```python
from build123d import *

# Parameters (mm, degrees)
F0_W     = 15.5
F0_H     = 15.5
F0_W_2   = 96
F0_H_2   = 44
F1_DEPTH = 5
F3_DEPTH = 5


with BuildPart() as f1:
    # F0 (on Top) → F1 (new body)
    with BuildSketch(Plane.XY):
        with BuildLine():
            ThreePointArc((0, 5), (1.464466, 1.464466), (5, 0))
            Line((5, 0), (105, 0))
            ThreePointArc((105, 0), (108.535534, 1.464466), (110, 5))
            Line((110, 5), (110, 170))
            ThreePointArc((110, 170), (108.535534, 173.535534), (105, 175))
            Line((105, 175), (5, 175))
            ThreePointArc((5, 175), (1.464466, 173.535534), (0, 170))
            Line((0, 170), (0, 5))
        make_face()
        with Locations((16.75, 16.75)):
            Rectangle(F0_W, F0_H, mode=Mode.SUBTRACT)
        with Locations((16.75, 42.25)):
            Rectangle(F0_W, F0_H, mode=Mode.SUBTRACT)
        with Locations((42.25, 16.75)):
            Rectangle(F0_W, F0_H, mode=Mode.SUBTRACT)
        with Locations((42.25, 42.25)):
            Rectangle(F0_W, F0_H, mode=Mode.SUBTRACT)
        with Locations((16.75, 67.75)):
            Rectangle(F0_W, F0_H, mode=Mode.SUBTRACT)
        with Locations((42.25, 67.75)):
            Rectangle(F0_W, F0_H, mode=Mode.SUBTRACT)
        with Locations((67.75, 16.75)):
            Rectangle(F0_W, F0_H, mode=Mode.SUBTRACT)
        with Locations((67.75, 42.25)):
            Rectangle(F0_W, F0_H, mode=Mode.SUBTRACT)
        with Locations((93.25, 16.75)):
            Rectangle(F0_W, F0_H, mode=Mode.SUBTRACT)
        with Locations((93.25, 42.25)):
            Rectangle(F0_W, F0_H, mode=Mode.SUBTRACT)
        with Locations((67.75, 67.75)):
            Rectangle(F0_W, F0_H, mode=Mode.SUBTRACT)
        with Locations((93.25, 67.75)):
            Rectangle(F0_W, F0_H, mode=Mode.SUBTRACT)
        with Locations((16.75, 93.25)):
            Rectangle(F0_W, F0_H, mode=Mode.SUBTRACT)
        with Locations((42.25, 93.25)):
            Rectangle(F0_W, F0_H, mode=Mode.SUBTRACT)
        with Locations((67.75, 93.25)):
            Rectangle(F0_W, F0_H, mode=Mode.SUBTRACT)
        with Locations((93.25, 93.25)):
            Rectangle(F0_W, F0_H, mode=Mode.SUBTRACT)
        with Locations((55, 138)):
            Rectangle(F0_W_2, F0_H_2, mode=Mode.SUBTRACT)
    extrude(amount=F1_DEPTH)

    # F2 (on face) → F3 (join)
    with BuildSketch(Plane.XY):
        with BuildLine():
            ThreePointArc((108, 168), (106.535534, 171.535534), (103, 173))
            Line((103, 173), (7, 173))
            ThreePointArc((7, 173), (3.464466, 171.535534), (2, 168))
            Line((2, 168), (2, 7))
            ThreePointArc((2, 7), (3.464466, 3.464466), (7, 2))
            Line((7, 2), (103, 2))
            ThreePointArc((103, 2), (106.535534, 3.464466), (108, 7))
            Line((108, 7), (108, 168))
        make_face()
        with BuildLine():
            Line((8, 172), (102, 172))
            ThreePointArc((102, 172), (105.535534, 170.535534), (107, 167))
            Line((107, 167), (107, 8))
            ThreePointArc((107, 8), (105.535534, 4.464466), (102, 3))
            Line((102, 3), (8, 3))
            ThreePointArc((8, 3), (4.464466, 4.464466), (3, 8))
            Line((3, 8), (3, 167))
            ThreePointArc((3, 167), (4.464466, 170.535534), (8, 172))
        make_face(mode=Mode.SUBTRACT)
    extrude(amount=-F3_DEPTH)


solid = f1.part
```
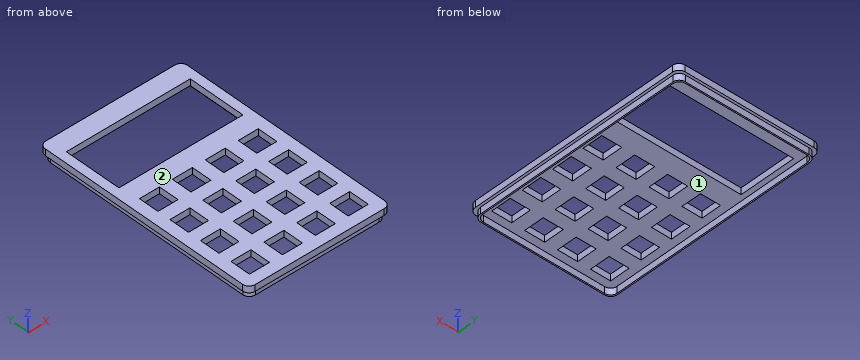
Source: CAD feature listing. Evaluate the final solid. Frame: model axes, mm. Face numbers are marked on the shaded views. Give positions to 0.01 mm unless a question says otherwise; leave off trailing zeros. Order: outer loops, then holes, each group sorted by start corner. A loop starts at its lowest first (then second) coordinate and runs counter-clockwise, first axis right, second up.
(1) Section query A-A (x = 30.5). Return the cut outline in (y, z).
(2) Section query D-D (y = 45). Return the cut outline in (x, z).
(3) Section query C-C (x = 67.5). State how many separate pieces and enclosed holes the cut face has, plus the area to 3 significant figures.
(4) Section query B-B (y = 151). Return the cut outline in (x, z), plus the area to 3 significant figures.
(5) Pull-direction query (X, two-part tool) for the marked faces 1 and 2; classes: +X half, -X half, draft (parallel to the pull), parting line (faces both ways), or undercut.
(6) Material intervals for line 1 along X through (y, z) = (96, 3.75); line 2 along Y through (x, z) = (68, 1.5); line 3 along X through (y, z) = (67, -4.5), sorted ascending.
(7) Contact query for flat-ended pins moving along their axis: P1, Ø1.5, axis at x = 38, y = 78, coming from the -Z side; P2, Ø4, axis at x = 98, y = 41.5, coming from the -Z side; P3, Ø1.5, axis at y = 56, z = -3.5, coming from the +X side. Output: stop coordinate, or through.
Outcome:
1. outline: (0, 0) - (2, 0) - (2, -5) - (3, -5) - (3, 0) - (116, 0) - (116, 5) - (0, 5) - close; (160, 0) - (172, 0) - (172, -5) - (173, -5) - (173, 0) - (175, 0) - (175, 5) - (160, 5) - close
2. outline: (0, 0) - (2, 0) - (2, -5) - (3, -5) - (3, 0) - (9, 0) - (9, 5) - (0, 5) - close; (24.5, 0) - (34.5, 0) - (34.5, 5) - (24.5, 5) - close; (50, 0) - (60, 0) - (60, 5) - (50, 5) - close; (75.5, 0) - (85.5, 0) - (85.5, 5) - (75.5, 5) - close; (101, 0) - (107, 0) - (107, -5) - (108, -5) - (108, 0) - (110, 0) - (110, 5) - (101, 5) - close
3. separate pieces: 6
3. enclosed holes: 0
3. area: 355 mm2
4. outline: (0, 0) - (2, 0) - (2, -5) - (3, -5) - (3, 0) - (7, 0) - (7, 5) - (0, 5) - close; (103, 0) - (107, 0) - (107, -5) - (108, -5) - (108, 0) - (110, 0) - (110, 5) - (103, 5) - close
4. area: 80.0 mm2
5. face 1: undercut
5. face 2: draft
6. line 1: x = 0 to 9, 24.5 to 34.5, 50 to 60, 75.5 to 85.5, 101 to 110
6. line 2: y = 0 to 9, 24.5 to 34.5, 50 to 60, 75.5 to 85.5, 101 to 116, 160 to 175
6. line 3: x = 2 to 3, 107 to 108
7. P1: stops at z = 0
7. P2: passes through
7. P3: stops at x = 108
